Part model, mm, in its own coordinate system. A direction names the side the tool comes from. Round coordinates to 2 decimals unless told otherwise and drop trailing zeros. Loops run counter-clockwise (first coordinate to the right, second up) from the corner with the lowest first, then second, coordinate; pieces in that order, holes last. Notation, with made-up numbers: (70.5, 81) -> (74.5, 81) arc R19 ccw to (74.5, 95) -> close; hole circle Ø4 at (53.5, -34.75). An arc over 180 degrees is marked (long way). Use a Markdown table: item, result. Add a question column.
Item 1: Probe line 1 (Z direction, x = 28, y = 3); line 2 (Z direction, x = 201, y = 4.8); line 3 (Z direction, x = 157.5, y = 4.15). List the from-to ranges inside material, lowest first. Write a range as [from, to].
Item 2: Cut at C-C, the plane x = 17. List the corners of the cut face in (y, z).
Item 3: Which spindle directions (+Z, -Z, +X, -X, +Y, -Y) get a long thin tool onto all of the face, cutting with end or side? Do faces 1 (the face through (18, 3, -134.493)), 2 (the face through (0, 3, -107)). Say none if no direction does.
Item 4: Cut at B-B, the plane z = -125.5. List the corners of the cut face in (x, y), plus the area to 3 significant figures.
Item 5: Cut at D-D, the plane y = 2.9. State how many separate pieces and enclosed holes the cut face has, plus the area to 3 significant figures.
Item 6: Cut at A-A, the plane x = 66.5. List the corners of the cut face in (y, z), plus the area to 3 significant figures.
Item 7: Flat gauge pins, fed straight in: pin 1 (2.5 mm diameter, centred on x = 13.5, y = 3, fed in from -Z); pin 2 (3 mm diameter, centred on y = 4.5, z = -179.5, fed in from +X); pin 3 (2.5 mm diameter, centred on x = 21, y = 2, fed in from +Z). Where does each tip first touch, or does it go through?
Item 8: Two-plate mould, pull along X, no slides. Class faces 3 (the face through (134.6, 2.7, -155.9)), 4 (the face through (28.17, 2.7, -27.37)), 5 (the face through (113, 3, -215.9)): pulls with the +X half, pulls with the -X half, needs draft (parallel to the pull), parting line crosses it, or undercut.
```python
from build123d import *

# Parameters (mm, degrees)
SKETCH1_W           = 228.6
SKETCH1_H           = 215.9
BOSS_EXTRUDE1_DEPTH = 5.334
CUT_EXTRUDE1_DEPTH  = 6.334
CIRPATTERN1_COUNT   = 4
SKETCH8_W           = 25.4
SKETCH8_H           = 5.334
CUT_EXTRUDE2_DEPTH  = 6.334
SKETCH11_R          = 1.524
CUT_EXTRUDE4_DEPTH  = 6.334
CUT_EXTRUDE5_DEPTH  = 6.334


with BuildPart() as part:
    # Sketch1 → Boss-Extrude1 (new body)
    with BuildSketch(Plane(origin=(0, 0, 0), x_dir=(1, 0, 0), z_dir=(0, 1, 0))):
        with Locations((114.3, 107.95)):
            Rectangle(SKETCH1_W, SKETCH1_H)
    extrude(amount=BOSS_EXTRUDE1_DEPTH)

    # Sketch6 → Cut-Extrude1 (cut, through all)
    with BuildSketch(Plane(origin=(0, 5.334, 0), x_dir=(1, 0, 0), z_dir=(0, 1, 0))):
        with BuildLine():
            Line((114.3, 165.1), (114.3, 160.02))
            ThreePointArc((114.3, 160.02), (134.911318287, 155.766926485), (152.155574853, 143.702487361))
            Line((152.155574853, 143.702487361), (155.848801668, 147.190534909))
            ThreePointArc((155.848801668, 147.190534909), (136.922178608, 160.431992483), (114.3, 165.1))
        make_face()
    cut_extrude1 = extrude(amount=-CUT_EXTRUDE1_DEPTH, mode=Mode.SUBTRACT)

    # CirPattern1: Cut-Extrude1 ×4 about axis
    cirpattern1_axis = Axis((114.20329472, 0, -107.72565), (0, 1, 0))
    for i in range(1, CIRPATTERN1_COUNT):
        add(cut_extrude1.rotate(cirpattern1_axis, i * 360 / CIRPATTERN1_COUNT), mode=Mode.SUBTRACT)

    # Sketch8 → Cut-Extrude2 (cut, through all)
    with BuildSketch(Plane(origin=(0, 5.334, 0), x_dir=(1, 0, 0), z_dir=(0, 1, 0))):
        with Locations((18.034, 131.826)):
            Rectangle(SKETCH8_W, SKETCH8_H)
        with Locations((210.566, 131.826)):
            Rectangle(SKETCH8_W, SKETCH8_H)
        with Locations((210.566, 84.074)):
            Rectangle(SKETCH8_W, SKETCH8_H)
        with Locations((18.034, 84.074)):
            Rectangle(SKETCH8_W, SKETCH8_H)
    extrude(amount=-CUT_EXTRUDE2_DEPTH, mode=Mode.SUBTRACT)

    # Sketch11 → Cut-Extrude4 (cut, through all)
    with BuildSketch(Plane(origin=(0, 5.334, 0), x_dir=(1, 0, 0), z_dir=(0, 1, 0))):
        with Locations((95.758, 6.604)):
            Circle(SKETCH11_R)
        with Locations((132.842, 6.604)):
            Circle(SKETCH11_R)
        with Locations((132.842, 43.688)):
            Circle(SKETCH11_R)
        with Locations((95.758, 43.688)):
            Circle(SKETCH11_R)
    extrude(amount=-CUT_EXTRUDE4_DEPTH, mode=Mode.SUBTRACT)

    # Sketch13 → Cut-Extrude5 (cut, through all)
    with BuildSketch(Plane(origin=(0, 5.334, 0), x_dir=(1, 0, 0), z_dir=(0, 1, 0))):
        Polygon((0, 215.9), (0, 161.925), (57.15, 215.9), align=None)
        Polygon((228.6, 161.925), (171.45, 215.9), (228.6, 215.9), align=None)
        Polygon((228.6, 0), (228.6, 53.975), (171.45, 0), align=None)
        Polygon((0, 53.975), (57.15, 0), (0, 0), align=None)
    extrude(amount=-CUT_EXTRUDE5_DEPTH, mode=Mode.SUBTRACT)


solid = part.part
```
A:
| question | item | result |
|---|---|---|
| 1 | line 1 | z = [-188.37, -134.49], [-129.16, -86.74], [-81.41, -27.53] |
| 1 | line 2 | z = [-187.99, -134.49], [-129.16, -86.74], [-81.41, -27.91] |
| 1 | line 3 | z = [-215.9, -78.37], [-70.07, 0] |
| 2 | outline | (0, -177.98) -> (5.33, -177.98) -> (5.33, -134.49) -> (0, -134.49) -> close; (0, -129.16) -> (5.33, -129.16) -> (5.33, -86.74) -> (0, -86.74) -> close; (0, -81.41) -> (5.33, -81.41) -> (5.33, -37.92) -> (0, -37.92) -> close |
| 3 | face 1 | +Y, -Y |
| 3 | face 2 | +Z, -Z, -X, +Y, -Y |
| 4 | outline | (0, 0) -> (59.63, 0) -> (59.63, 5.33) -> (0, 5.33) -> close; (65, 0) -> (228.6, 0) -> (228.6, 5.33) -> (65, 5.33) -> close |
| 4 | area | 1,190 mm^2 |
| 5 | separate pieces | 1 |
| 5 | enclosed holes | 12 |
| 5 | area | 41,700 mm^2 |
| 6 | outline | (0, -215.9) -> (5.33, -215.9) -> (5.33, -139.63) -> (0, -139.63) -> close; (0, -129.2) -> (5.33, -129.2) -> (5.33, 0) -> (0, 0) -> close |
| 6 | area | 1,100 mm^2 |
| 7 | pin 1 | stops at z = -175.86 |
| 7 | pin 2 | stops at x = 211.58 |
| 7 | pin 3 | stops at z = -32.96 |
| 8 | face 3 | undercut |
| 8 | face 4 | pulls with the -X half |
| 8 | face 5 | needs draft |
